```python
from build123d import *

# Parameters (mm, degrees)
PAD_DEPTH   = 85
FILLET_R    = 10
FILLET001_R = 4


with BuildPart() as part:
    # Sketch → Pad (new body)
    with BuildSketch(Plane.XY):
        Polygon((0, 20), (0, 0), (20, 0), (20, 5), (5, 5), (5, 20), align=None)
    extrude(amount=PAD_DEPTH)

    # Fillet
    fillet_edges = [part.edges().sort_by_distance(p)[0] for p in [
        (0, 0, 42.5),
    ]]
    fillet(fillet_edges, radius=FILLET_R)

    # Fillet001
    fillet001_edges = [part.edges().sort_by_distance(p)[0] for p in [
        (0, 20, 42.5),
        (20, 0, 42.5),
    ]]
    fillet(fillet001_edges, radius=FILLET001_R)


solid = part.part
```
For this review, take the finished solid that the model builds, in its own axes (mm). A direction names the side the tool comes from. Coordinates: 2 decimals unless noted, no trailing zeros. Write each loop counter-clockwise with the first axis right and the second up, starting at its lowest first coordinate (ties: lowest second). Pieces come first, ordered by that corner, then holes.
(1) Add section B-B on x = 13.5. Give the boundary of the cut face in (y, z), then the cut area to 3 significant figures.
(2) Wall thickness on probe 1 along X at (y, z) = (13, 77.5); probe 2 along X at (y, z) = (1.25, 39): over which ranges is each line inside the solid? List them lowest first.
(3) Add section A-A on z = 79. Give the boundary of the cut face in (x, y), then the cut area to 3 significant figures.
(4) For pin 1 Ø1.5 at (x, z) = (3, 69.5) entering from -Y; pin 2 Ø3 at (y, z) = (7, 58.5) entering from +X; pin 3 Ø4 at (x, z) = (5, 26.5) entering from -Y, all flat-tipped, find the tip position at first contact; note any pin that passes through.
(5) Tool access review of faces 1 (the face through (1.141, 18.797, 43.095)), 2 (the face through (13, 5, 42)): name each direction out of +Z, -Z, +X, -X, +Y, -Y from which nothing blocks a thin tool from reaching the whole face with its end or side.
Answer sheet:
1. outline: (0, 0) - (5, 0) - (5, 85) - (0, 85) - close
1. area: 425 mm2
2. probe 1: x = 0 to 5
2. probe 2: x = 5.16 to 18.9
3. outline: (0, 10) arc R10 ccw to (10, 0) - (16, 0) arc R4 ccw to (20, 4) - (20, 5) - (5, 5) - (5, 20) - (4, 20) arc R4 ccw to (0, 16) - close
3. area: 147 mm2
4. pin 1: stops at y = 2.19
4. pin 2: stops at x = 5
4. pin 3: stops at y = 0.46
5. face 1: +Z, -Z, -X, +Y
5. face 2: +Z, -Z, +X, +Y
